Part model, mm, in its own coordinate system. Coordinates: 2 decimals unless noted, no trailing zeros. Order: outer loops, then holes, each group sorted by start corner. A loop starts at its lowest first (then second) coordinate and runs counter-clockwise, first axis right, second up. Notation, with made-up numbers: M 30,39 L 54,39 A7 ccw 54,50 Z; hole C 16,1.5 d9. An arc over 180 degrees is marked long. Write item = value, one per line. Start each with the question number.
from build123d import *

# Parameters (mm, degrees)
F0_W     = 50
F0_H     = 50
F1_DEPTH = 50
F5_DEPTH = 60
F6_DEPTH = 60
F7_DEPTH = 60


with BuildPart() as f1:
    # F0 (on Top) → F1 (new body)
    with BuildSketch(Plane.XY):
        Rectangle(F0_W, F0_H)
    extrude(amount=F1_DEPTH)

    # F2 (on face) → F5 (cut)
    with BuildSketch(Plane.XZ.offset(25)):
        with BuildLine():
            ThreePointArc((2.61e-08, 50), (17.6776695389, 42.6776695204), (25, 25))
            Line((25, 25), (25, 50))
            Line((25, 50), (2.61e-08, 50))
        make_face()
        with BuildLine():
            Line((25, 0), (25, 25))
            ThreePointArc((25, 25), (17.677669509, 7.3223304497), (-5.83e-08, 0))
            Line((-5.83e-08, 0), (25, 0))
        make_face()
        with BuildLine():
            Line((-25, 0), (-5.83e-08, 0))
            ThreePointArc((-5.83e-08, 0), (-17.6776695503, 7.322330491), (-25, 25))
            Line((-25, 25), (-25, 0))
        make_face()
        with BuildLine():
            ThreePointArc((-25, 25), (-17.6776695204, 42.6776695389), (2.61e-08, 50))
            Line((2.61e-08, 50), (-25, 50))
            Line((-25, 50), (-25, 25))
        make_face()
    extrude(amount=-F5_DEPTH, mode=Mode.SUBTRACT)

    # F4 (on face) → F6 (cut)
    with BuildSketch(Plane.YZ.offset(25)):
        with BuildLine():
            ThreePointArc((-25, 25), (-17.6776695204, 42.6776695389), (2.61e-08, 50))
            Line((2.61e-08, 50), (-25, 50))
            Line((-25, 50), (-25, 25))
        make_face()
        with BuildLine():
            ThreePointArc((2.61e-08, 50), (17.6776695389, 42.6776695204), (25, 25))
            Line((25, 25), (25, 50))
            Line((25, 50), (2.61e-08, 50))
        make_face()
        with BuildLine():
            Line((25, 0), (25, 25))
            ThreePointArc((25, 25), (17.677669509, 7.3223304497), (-5.83e-08, 0))
            Line((-5.83e-08, 0), (25, 0))
        make_face()
        with BuildLine():
            Line((-25, 0), (-5.83e-08, 0))
            ThreePointArc((-5.83e-08, 0), (-17.6776695503, 7.322330491), (-25, 25))
            Line((-25, 25), (-25, 0))
        make_face()
    extrude(amount=-F6_DEPTH, mode=Mode.SUBTRACT)

    # F3 (on face) → F7 (cut)
    with BuildSketch(Plane.XY.offset(50)):
        with BuildLine():
            Line((25, -25), (25, 0))
            ThreePointArc((25, 0), (17.677669509, -17.6776695503), (-5.83e-08, -25))
            Line((-5.83e-08, -25), (25, -25))
        make_face()
        with BuildLine():
            Line((-25, -25), (-5.83e-08, -25))
            ThreePointArc((-5.83e-08, -25), (-17.6776695595, -17.6776694998), (-25, 2.61e-08))
            Line((-25, 2.61e-08), (-25, -25))
        make_face()
        with BuildLine():
            ThreePointArc((-25, 2.61e-08), (-17.6776695204, 17.6776695389), (0, 25))
            Line((0, 25), (-25, 25))
            Line((-25, 25), (-25, 2.61e-08))
        make_face()
        with BuildLine():
            ThreePointArc((0, 25), (17.6776695297, 17.6776695297), (25, 0))
            Line((25, 0), (25, 25))
            Line((25, 25), (0, 25))
        make_face()
    extrude(amount=-F7_DEPTH, mode=Mode.SUBTRACT)


solid = f1.part
Item 1: Cut at D-D, the plane x = 19. Write the cut outline in (y, z), and give its area (3 significant figures).
Item 2: Cut at C-C, the plane z = 4.5. Write the cut outline in (x, y), and give its area (3 significant figures).
Item 3: Cut at A-A, the plane x = -1. Write the cut outline in (y, z).
Item 4: Wall check: line 1 along Y through (x, z) = (2, 40); line 2 along X through (y, z) = (-8.5, 30.5); line 3 along Z through (x, y) = (-10.5, -2). Give the ranges that are in metal, low to high. Write a range as [from, to].
Item 5: Flat gauge pins, fed straight in: pin 1 (12 mm diameter, centred on y = 11, z = 13, fed in from -X); pin 2 (2 mm diameter, centred on x = 19.5, y = -8.5, fed in from +Z); pin 3 (5 mm diameter, centred on x = 15.5, y = 17, fed in from +Z). Where does each tip first touch, or does it go through?
Filled sheet:
q1.outline = M -16.25,8.75 L 16.25,8.75 L 16.25,41.25 L -16.25,41.25 Z
q1.area = 1,060 mm2
q2.outline = M -14.31,-14.31 L 14.31,-14.31 L 14.31,14.31 L -14.31,14.31 Z
q2.area = 819 mm2
q3.outline = M -24.98,24 A25 ccw -1,0.02 L 1,0.02 A25 ccw 24.98,24 L 24.98,26 A25 ccw 1,49.98 L -1,49.98 A25 ccw -24.98,26 Z
q4.line_1 = [-20, 20]
q4.line_2 = [-23.51, 23.51]
q4.line_3 = [2.31, 47.69]
q5.pin_1 = -23.91
q5.pin_2 = 41.82
q5.pin_3 = 45.26
